For this review, take the finished solid that the model builds, in its own axes (mm). A direction names the side the tool comes from. Coordinates: 2 decimals unless noted, no trailing zeros. Loops run counter-clockwise (first coordinate to the right, second up) from the corner with the lowest first, then second, coordinate; pieces in that order, holes last. Notation, with made-up numbers: (-19, 40.25) - (32, 40.25) arc R19 ccw to (32, 66.25) - close; hole circle Ø11 at (24.5, 46.25). An arc over 180 degrees is marked (long way). One line per item, written item: value. Start each with the question number.
1. Take a section at D-D, the plane y = -18. State the section outline as (x, z) points, and give its area (3 significant figures).
2. Take a section at A-A, the plane x = 0. State the section outline as (y, z) points, and give its area (3 significant figures).
3. For faces 4 (the face through (2.2, 9, 3.3)), 5 (the face through (-6, -10, 6)), 6 (the face through (17.605, -17.803, 3.944)), list the 3-axis set-ups (+Z, -Z, +X, -X, +Y, -Y) from which the entire face can be reached by the end or side of a thin tool; tool diameter is ignored.
4. The part is to be moulded in two halves that separate along Y. For faces 1 (the face through (6, -10, 6)), 2 (the face through (-23.247, -19.857, 3.944)), 3 (the face through (-9.01, -27.15, 5.46)), say which applies: released by +Y, released by -Y, zero draft, split by the parting line, or undercut.
5. Take a section at C-C, the plane z = 5.25. State the section outline as (x, y) points, and give its area (3 significant figures).
6. Take a section at B-B, the plane y = 10. State the section outline as (x, z) points, and give its area (3 significant figures).
7. Insertion check: pin 1 (11.5 mm diameter, centred on x = 0, y = 10, fed in from +Z); pin 2 (3.5 mm diameter, centred on x = 0, y = 10, fed in from -Z); pin 3 (4 mm diameter, centred on x = 0.5, z = 6.5, fed in from -Y). Each pin has a flat end and moves straight along its axis. Give the tip position at first contact, or say it passes through.
8. To check wall thickness, follow line 1 (Y direction, x = 0, z = 5.8); line 2 (X direction, y = -9.5, z = 4); line 3 (Y direction, x = 20, z = 3). State the ranges of each line that lie inside material, in increasing order. Write a range as from..to.
```python
from build123d import *

# Parameters (mm, degrees)
SKETCH_1_R          = 5
SKETCH_1_R_2        = 3.25
SKETCH_1_R_3        = 2.25
EXTRUDE_1_DEPTH     = 8
SKETCH_1_3_R        = 5
SKETCH_1_3_R_2      = 2.25
CUT_EXTRUDE_1_DEPTH = 3.3
SKETCH_2_W          = 12
SKETCH_2_H          = 30
CUT_EXTRUDE_2_DEPTH = 5
FILLET_1_R          = 10


with BuildPart() as part:
    # Sketch 1 → Extrude 1 (new body)
    # profile 1 of 2: a face of its own
    with BuildSketch(Plane.XY):
        with BuildLine():
            Line((30, 30), (-30, 30))
            ThreePointArc((-30, 30), (-37.071067812, 27.071067812), (-40, 20))
            Line((-40, 20), (-40, -20))
            ThreePointArc((-40, -20), (-37.071067812, -27.071067812), (-30, -30))
            Line((-30, -30), (30, -30))
            ThreePointArc((30, -30), (37.071067812, -27.071067812), (40, -20))
            Line((40, -20), (40, 20))
            ThreePointArc((40, 20), (37.071067812, 27.071067812), (30, 30))
        make_face()
        with Locations((0, 10)):
            Circle(SKETCH_1_R, mode=Mode.SUBTRACT)
        with Locations((-20, -20)):
            Circle(SKETCH_1_R_2, mode=Mode.SUBTRACT)
        with Locations((20, -20)):
            Circle(SKETCH_1_R_2, mode=Mode.SUBTRACT)
    # profile 2 of 2: a face of its own
    with BuildSketch(Plane.XY):
        with Locations((0, 10)):
            Circle(SKETCH_1_R)
        with Locations((0, 10)):
            Circle(SKETCH_1_R_3, mode=Mode.SUBTRACT)
    extrude(amount=EXTRUDE_1_DEPTH)

    # Sketch 1_3 → Cut-Extrude 1 (cut)
    with BuildSketch(Plane.XY):
        with Locations((0, 10)):
            Circle(SKETCH_1_3_R)
        with Locations((0, 10)):
            Circle(SKETCH_1_3_R_2, mode=Mode.SUBTRACT)
    extrude(amount=CUT_EXTRUDE_1_DEPTH, mode=Mode.SUBTRACT)

    # Sketch 2 → Cut-Extrude 2 (cut)
    with BuildSketch(Plane.XY.offset(8)):
        with Locations((0, -15)):
            Rectangle(SKETCH_2_W, SKETCH_2_H)
    extrude(amount=-CUT_EXTRUDE_2_DEPTH, mode=Mode.SUBTRACT)

    # Fillet 1
    fillet_1_edges = [part.edges().sort_by_distance(p)[0] for p in [
        (6, -30, 5.5),
        (-6, -30, 5.5),
    ]]
    fillet(fillet_1_edges, radius=FILLET_1_R)


solid = part.part
```
Solutions:
1. outline: (-40, 0) - (-22.56, 0) - (-22.56, 8) - (-40, 8) - close; (-17.44, 0) - (17.44, 0) - (17.44, 8) - (6, 8) - (6, 3) - (-6, 3) - (-6, 8) - (-17.44, 8) - close; (22.56, 0) - (40, 0) - (40, 8) - (22.56, 8) - close
1. area: 498 mm2
2. outline: (-30, 0) - (5, 0) - (5, 3.3) - (7.75, 3.3) - (7.75, 8) - (0, 8) - (0, 3) - (-30, 3) - close; (12.25, 3.3) - (15, 3.3) - (15, 0) - (30, 0) - (30, 8) - (12.25, 8) - close
2. area: 276 mm2
3. face 4: -Z
3. face 5: +Z, -Y
3. face 6: +Z, -Z
4. face 1: zero draft
4. face 2: undercut
4. face 3: released by -Y
5. outline: (-40, -20) arc R10 ccw to (-30, -30) - (-16, -30) arc R10 ccw to (-6, -20) - (-6, 0) - (6, 0) - (6, -20) arc R10 ccw to (16, -30) - (30, -30) arc R10 ccw to (40, -20) - (40, 20) arc R10 ccw to (30, 30) - (-30, 30) arc R10 ccw to (-40, 20) - close; hole circle Ø6.5 at (-20, -20); hole circle Ø4.5 at (0, 10); hole circle Ø6.5 at (20, -20)
5. area: 4,230 mm2
6. outline: (-40, 0) - (-5, 0) - (-5, 3.3) - (-2.25, 3.3) - (-2.25, 8) - (-40, 8) - close; (2.25, 3.3) - (5, 3.3) - (5, 0) - (40, 0) - (40, 8) - (2.25, 8) - close
6. area: 586 mm2
7. pin 1: z = 8
7. pin 2: through
7. pin 3: y = 0
8. line 1: 0..7.75, 12.25..30
8. line 2: -40..-6, 6..40
8. line 3: -30..-23.25, -16.75..30
